The model under review builds one solid part; all positions refer to its coordinate system, in mm. A direction names the side the tool comes from. Round coordinates to 2 decimals unless told otherwise and drop trailing zeros. Loops run counter-clockwise (first coordinate to the right, second up) from the corner with the lowest first, then second, coordinate; pieces in that order, holes last. Notation, with made-up numbers: M 77,37.25 L 93,37.25 A24 ccw 93,47.25 Z; hole C 55,-26.5 d6. An arc over 180 degrees is marked long. Use a Markdown table: item, result. Add a question column.
```python
from build123d import *

# Parameters (mm, degrees)
SKETCH1_W           = 40
SKETCH1_H           = 30
BOSS_EXTRUDE1_DEPTH = 20
SKETCH2_R           = 3.15
SKETCH2_W           = 16
SKETCH2_H           = 15
CUT_EXTRUDE1_DEPTH  = 20
SKETCH3_W           = 10
SKETCH3_H           = 5
BOSS_EXTRUDE2_DEPTH = 10
FILLET3_R           = 5
FILLET4_R           = 5
SKETCH6_R           = 3
CUT_EXTRUDE3_DEPTH  = 140
FILLET5_R           = 10
FILLET6_R           = 5
FILLET7_R           = 7


with BuildPart() as part:
    # Sketch1 → Boss-Extrude1 (new body)
    with BuildSketch(Plane(origin=(0, 0, 0), x_dir=(1, 0, 0), z_dir=(0, 1, 0))):
        with Locations((20, 15)):
            Rectangle(SKETCH1_W, SKETCH1_H)
    extrude(amount=BOSS_EXTRUDE1_DEPTH)

    # Sketch2 → Cut-Extrude1 (cut)
    with BuildSketch(Plane(origin=(0, 20, 0), x_dir=(1, 0, 0), z_dir=(0, 1, 0))):
        with Locations(Location((10, 23, 0), (0, 0, 270))):
            Circle(SKETCH2_R)
        with Locations(Location((30, 23, 0), (0, 0, 270))):
            Circle(SKETCH2_R)
        with Locations((20.029547187, 7.5)):
            Rectangle(SKETCH2_W, SKETCH2_H)
    extrude(amount=-CUT_EXTRUDE1_DEPTH, mode=Mode.SUBTRACT)

    # Sketch3 → Boss-Extrude2 (add)
    with BuildSketch(Plane(origin=(0, 0, -30), x_dir=(-1, 0, 0), z_dir=(0, 0, -1))):
        with Locations((-20, 17.5)):
            Rectangle(SKETCH3_W, SKETCH3_H)
    extrude(amount=BOSS_EXTRUDE2_DEPTH)

    # Fillet3
    fillet3_edges = [part.edges().sort_by_distance(p)[0] for p in [
        (25, 17.5, -30),
        (15, 17.5, -30),
    ]]
    fillet(fillet3_edges, radius=FILLET3_R)

    # Fillet4
    fillet4_edges = [part.edges().sort_by_distance(p)[0] for p in [
        (20, 15, -30),
    ]]
    fillet(fillet4_edges, radius=FILLET4_R)

    # Sketch6 → Cut-Extrude3 (cut)
    with BuildSketch(Plane.ZY):
        with Locations((-6, 10)):
            Circle(SKETCH6_R)
    extrude(amount=-CUT_EXTRUDE3_DEPTH, mode=Mode.SUBTRACT)

    # Fillet5
    fillet5_edges = [part.edges().sort_by_distance(p)[0] for p in [
        (34.014773594, 20, 0),
        (34.014773594, 0, 0),
        (6.014773594, 0, 0),
        (6.014773594, 20, 0),
    ]]
    fillet(fillet5_edges, radius=FILLET5_R - 0.0001)  # a hair under: the kernel refuses the full size

    # Fillet6
    fillet6_edges = [part.edges().sort_by_distance(p)[0] for p in [
        (25, 17.5, -40),
        (15, 17.5, -40),
    ]]
    fillet(fillet6_edges, radius=FILLET6_R - 0.0001)  # a hair under: the kernel refuses the full size

    # Fillet7
    fillet7_edges = [part.edges().sort_by_distance(p)[0] for p in [
        (0, 10, -30),
        (40, 10, -30),
    ]]
    fillet(fillet7_edges, radius=FILLET7_R)


solid = part.part
```
(1) Consider section C-C, the plane y = 18.75. Give the number of separate pieces and of enclosed holes in the cut face, then the cut area to 3 significant figures.
(2) For faces 1 (the face through (13.123, 10.14, -23.41)), 2 (the face through (20, 15, -37)), list the 3-axis set-ups (+Z, -Z, +X, -X, +Y, -Y) from which the entire face can be reached by the end or side of a thin tool; tool diameter is ignored.
(3) Insertion check: pin 1 Ø5 at (x, y) = (34, 6.5) entering from -Z; pin 2 Ø5 at (x, z) = (28.5, -4) entering from +Y; pin 3 Ø5 at (x, y) = (16.5, 15.5) entering from -Z. Each pin has a flat end and moves straight along its axis. Give the tip position at first contact, or say it passes through.
(4) Consider section B-B, the plane y = 8.75. Give the boundary of the cut face in (x, z), then the cut area to 3 significant figures.
(5) Draft analysis for pull direction Y (two halves, no side actions). For faces 3 (the face through (34.1, 2.85, -3.01)), 4 (the face through (33.93, 10.9, -3.14)), 5 (the face through (28.03, 10, -11)), state which applies: released by +Y, released by -Y, zero draft, split by the parting line, or undercut.
(6) To check wall thickness, follow probe 1 along X at (y, z) = (10.75, -23); probe 2 along X at (y, z) = (8.5, -10); probe 3 along X at (y, z) = (7.25, -24). State the ranges of each line that lie inside material, in increasing order.
(7) Consider section A-A, the plane z = -13. Give the boundary of the cut face in (x, y).
Found:
| question | item | result |
|---|---|---|
| 1 | separate pieces | 1 |
| 1 | enclosed holes | 2 |
| 1 | area | 853 mm^2 |
| 2 | face 1 | +Y, -Y |
| 2 | face 2 | -Z, +X, -X, -Y |
| 3 | pin 1 | stops at z = -30 |
| 3 | pin 2 | stops at y = 19.37 |
| 3 | pin 3 | stops at z = -39.9 |
| 4 | outline | M 0,-23 A7 ccw 7,-30 L 33,-30 A7 ccw 40,-23 L 40,-8.73 L 28.03,-8.73 L 28.03,-15 L 12.03,-15 L 12.03,-8.73 L 0,-8.73 Z; M 0,-3.27 L 12.03,-3.27 L 12.03,-0.08 L 0,-0.08 Z; M 28.03,-3.27 L 40,-3.27 L 40,-0.08 L 28.03,-0.08 Z; hole C 10,-23 d6.3; hole C 30,-23 d6.3 |
| 4 | area | 744 mm^2 |
| 5 | face 3 | released by -Y |
| 5 | face 4 | undercut |
| 5 | face 5 | zero draft |
| 6 | probe 1 | x = 0 to 6.85, 13.15 to 26.85, 33.15 to 40 |
| 6 | probe 2 | x = 0 to 12.03, 28.03 to 40 |
| 6 | probe 3 | x = 0.07 to 7.01, 12.99 to 27.01, 32.99 to 39.93 |
| 7 | outline | M 0,0 L 12.03,0 L 12.03,20 L 0,20 Z; M 28.03,0 L 40,0 L 40,20 L 28.03,20 Z |
